Here's how the part is built. I have some questions about the finished solid (model axes, mm). Face numbers are marked on the shaded views. A direction names the side the tool comes from. Coordinates: 2 decimals unless noted, no trailing zeros. Write each loop counter-clockwise with the first axis right and the second up, starting at its lowest first coordinate (ties: lowest second). Pieces come first, ordered by that corner, then holes. Notation, with made-up numbers: (-31.75, 19) -> (6.25, 19) arc R17 cw to (6.25, 40) -> close; hole circle Ø11 at (-33.5, -9). An arc over 180 degrees is marked (long way). Use a Markdown table: item, result. Add a question column.
Item 1: Imagine slicing it at D-D, the plane y = -66.5. Write out the boundary of the cut face in (x, z).
Item 2: Imagine slicing it at A-A, the plane x = 4. Write out the boundary of the cut face in (y, z).
Item 3: If I drill on line 1 along X through (y, z) = (-89, 5.25); line 2 along X through (y, z) = (-97, 0.4) (3 decimals), over which ranges is the centre line in solid material (lowest first)? Write a range as from..to.
Item 4: On a 3-axis mill with a long thin cutter (end or side, diameter ignored), from which of +Z, -Z, +X, -X, +Y, -Y can I reach the whole of each face in a straight line? I mean the marked faces 1 and 2. Say none if no direction works.
Item 5: If we mould it in two halves opening along Z, with no side actions, what happens to the marked faces 3, 4 and 5? For each: pulls with the +Z half, pulls with the -Z half, needs draft (parallel to the pull), parting line crosses it, or undercut.
Item 6: Imagine slicing it at B-B, the plane z = 11. Write out the boundary of the cut face in (x, y).
Item 7: Imagine slicing it at C-C, the plane y = -15. Write out the boundary of the cut face in (x, z) (3 decimals), and give its area (3 significant figures).
```python
from build123d import *

# Parameters (mm, degrees)
F0_W     = 13.85
F0_H     = 13.85
F1_DEPTH = 100
F2_T     = -0.8
F3_R     = 1.5
F4_DEPTH = 25


with BuildPart() as f1:
    # F0 (on Front) → F1 (new body)
    with BuildSketch(Plane.XZ):
        with Locations((6.925, 6.925)):
            Rectangle(F0_W, F0_H)
    extrude(amount=F1_DEPTH)

    # F2
    f2_openings = [f1.faces().sort_by_distance(p)[0] for p in [
        (6.925, -100, 6.925),
        (6.925, 0, 6.925),
    ]]
    offset(amount=F2_T, openings=f2_openings)

    # F3 (on face) → F4 (cut)
    with BuildSketch(Plane.XY.offset(13.85)):
        with Locations((6.925, -97)):
            Circle(F3_R)
        with Locations((6.925, -85)):
            Circle(F3_R)
        with Locations((6.925, -15)):
            Circle(F3_R)
        with Locations((6.925, -3)):
            Circle(F3_R)
    extrude(amount=-F4_DEPTH, mode=Mode.SUBTRACT)


solid = f1.part
```
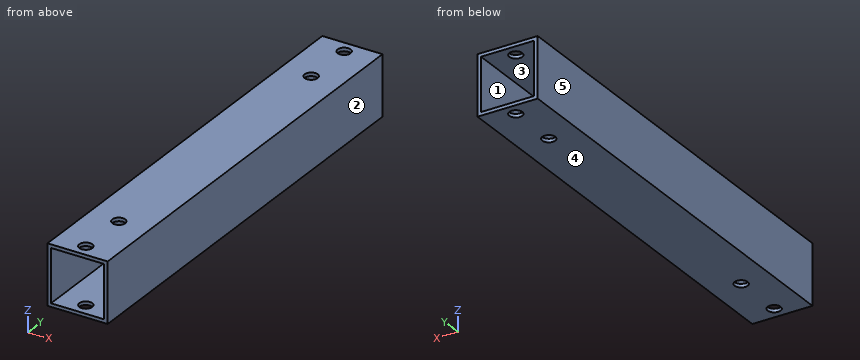
Ans:
| question | item | result |
|---|---|---|
| 1 | outline | (0, 0) -> (13.85, 0) -> (13.85, 13.85) -> (0, 13.85) -> close; hole (0.8, 0.8) -> (13.05, 0.8) -> (13.05, 13.05) -> (0.8, 13.05) -> close |
| 2 | outline | (-100, 0) -> (0, 0) -> (0, 0.8) -> (-100, 0.8) -> close; (-100, 13.05) -> (0, 13.05) -> (0, 13.85) -> (-100, 13.85) -> close |
| 3 | line 1 | x = 0..0.8, 13.05..13.85 |
| 3 | line 2 | x = 0..5.425, 8.425..13.85 |
| 4 | face 1 | +Y, -Y |
| 4 | face 2 | +Z, -Z, +X, +Y, -Y |
| 5 | face 3 | undercut |
| 5 | face 4 | pulls with the -Z half |
| 5 | face 5 | needs draft |
| 6 | outline | (0, -100) -> (0.8, -100) -> (0.8, 0) -> (0, 0) -> close; (13.05, -100) -> (13.85, -100) -> (13.85, 0) -> (13.05, 0) -> close |
| 7 | outline | (0, 0) -> (5.425, 0) -> (5.425, 0.8) -> (0.8, 0.8) -> (0.8, 13.05) -> (5.425, 13.05) -> (5.425, 13.85) -> (0, 13.85) -> close; (8.425, 0) -> (13.85, 0) -> (13.85, 13.85) -> (8.425, 13.85) -> (8.425, 13.05) -> (13.05, 13.05) -> (13.05, 0.8) -> (8.425, 0.8) -> close |
| 7 | area | 37.0 mm^2 |
